from build123d import *

# Parameters (mm, degrees)
SKETCH_1_W          = 130
SKETCH_1_H          = 90
EXTRUDE_1_DEPTH     = 1.5
SKETCH_2_R          = 4
CUT_EXTRUDE_1_DEPTH = 1.5
FILLET_1_R          = 2


with BuildPart() as part:
    # ｽｹｯﾁ1 → ﾎﾞｽ - 押し出し1 (new body)
    with BuildSketch(Plane.XY):
        Rectangle(SKETCH_1_W, SKETCH_1_H)
    extrude(amount=EXTRUDE_1_DEPTH)

    # ｽｹｯﾁ2 → ｶｯﾄ - 押し出し1 (cut)
    with BuildSketch(Plane.XY.offset(1.5)):
        with Locations((-40, 0)):
            Circle(SKETCH_2_R)
        with Locations(Location((40, 0, 0), (0, 0, 180))):
            Circle(SKETCH_2_R)
    extrude(amount=-CUT_EXTRUDE_1_DEPTH, mode=Mode.SUBTRACT)

    # ﾌｨﾚｯﾄ1
    fillet_1_edges = [part.edges().sort_by_distance(p)[0] for p in [
        (65, -45, 0.75),
        (-65, -45, 0.75),
        (-65, 45, 0.75),
        (65, 45, 0.75),
    ]]
    fillet(fillet_1_edges, radius=FILLET_1_R)


solid = part.part
CAD build for the part. Positions are in the model's coordinates, mm. Round coordinates to 2 decimals unless told otherwise and drop trailing zeros. Loops run counter-clockwise (first coordinate to the right, second up) from the corner with the lowest first, then second, coordinate; pieces in that order, holes last. Notation, with made-up numbers: M -33.5,71.25 L -14.5,71.25 A14 ccw -14.5,75.25 Z; hole C 7.5,-23 d1. An arc over 180 degrees is marked long. One line per question, with ' | ' between items. Start each with the question number.
Item 1: Two-plate mould, pull along Y, no slides. Class faces 1 (the cylindrical face through (-43.2, -2.4, 0.8)), 2 (the flat face through (-1, 1, 1.5)): pulls with the +Y half, pulls with the -Y half, needs draft (parallel to the pull), parting line crosses it, or undercut.
Item 2: Pin check, flat tip, straight feed: pin 1 Ø5 at (x, y) = (-40, 0) entering from +Z. Stop position of the tip, or through.
Item 3: Cut at A-A, the plane x = -40. Write the cut outline in (y, z).
Item 4: Cut at B-B, the plane y = 0. Write the cut outline in (x, z), plus the area to 3 significant figures.
Item 5: Wall check: line 1 (Y direction, x = 40, z = 0.65). Give the ranges that are in metal, low to high.
Responses:
1) face 1: undercut | face 2: needs draft
2) pin 1: passes through
3) outline: M -45,0 L -4,0 L -4,1.5 L -45,1.5 Z; M 4,0 L 45,0 L 45,1.5 L 4,1.5 Z
4) outline: M -65,0 L -44,0 L -44,1.5 L -65,1.5 Z; M -36,0 L 36,0 L 36,1.5 L -36,1.5 Z; M 44,0 L 65,0 L 65,1.5 L 44,1.5 Z | area: 171 mm²
5) line 1: y = -45 to -4, 4 to 45
